from build123d import *

# Parameters (mm, degrees)
F1_DEPTH = 63.5
F2_DEPTH = 25.4
F3_DEPTH = 7.9375
F5_R     = 6.35
F6_R     = 9.6111188935
F7_DEPTH = 85.726


with BuildPart() as f1:
    # F0 (on Front) → F1 (new body, symmetric)
    with BuildSketch(Plane.XZ):
        Polygon((-41.275, 9.525), (-41.275, -9.525), (41.275, -9.525), (41.275, 9.525), (22.225, 9.525), align=None)
    extrude(amount=F1_DEPTH, both=True)

    # F0 (on Front) → F2 (join, symmetric)
    with BuildSketch(Plane.XZ):
        with BuildLine():
            Line((22.225, 9.525), (41.275, 9.525))
            Line((41.275, 9.525), (41.275, 36.5252))
            ThreePointArc((41.275, 36.5252), (45.9246798487, 47.7505201513), (57.15, 52.4002))
            Line((57.15, 52.4002), (60.325, 52.4002))
            Line((60.325, 52.4002), (60.325, 71.4502))
            Line((60.325, 71.4502), (57.15, 71.4502))
            add(Edge.make_bspline(
                [(53.2220163185, 71.2286086107), (54.5371358708, 71.3237902727), (55.8469463929, 71.3977482988), (57.15, 71.4502)],
                knots=[112.6539740509, 112.6539740509, 112.6539740509, 112.6539740509, 116.2850421165, 116.2850421165, 116.2850421165, 116.2850421165], degree=3))
            ThreePointArc((53.2220163185, 71.2286086107), (31.1025389426, 59.790740988), (22.225, 36.5252))
            Line((22.225, 36.5252), (22.225, 9.525))
        make_face()
        Polygon((85.725, 71.4502), (60.325, 71.4502), (60.325, 52.4002), (85.725, 52.4002), (85.725, 61.9125), align=None)
    extrude(amount=F2_DEPTH, both=True)

    # F0 (on Front) → F3 (join, symmetric)
    with BuildSketch(Plane.XZ):
        with BuildLine():
            add(Edge.make_bspline(
                [(-41.275, 9.525), (-33.4914332719, 44.8937261862), (12.4204005857, 68.2755952564), (53.2220163185, 71.2286086107)],
                knots=[0, 0, 0, 0, 112.6539740509, 112.6539740509, 112.6539740509, 112.6539740509], degree=3))
            Line((-41.275, 9.525), (22.225, 9.525))
            Line((22.225, 9.525), (22.225, 36.5252))
            ThreePointArc((22.225, 36.5252), (31.1025389426, 59.790740988), (53.2220163185, 71.2286086107))
        make_face()
    extrude(amount=F3_DEPTH, both=True)

    # F0 (on Front) → F4 (revolve)
    with BuildSketch(Plane.XZ):
        Polygon((85.725, 76.2), (85.725, 71.4502), (85.725, 61.9125), (85.725, 52.4002), (85.725, 47.625), (111.125, 47.625), (111.125, 76.2), align=None)
    revolve(axis=Axis((85.725, 0, 69.05625), (0, 0, 1)))

    # F5
    f5_edges = [f1.edges().sort_by_distance(p)[0] for p in [
        (41.275, -63.5, 0),
        (-41.275, -63.5, 0),
        (41.275, 63.5, 0),
        (-41.275, 63.5, 0),
    ]]
    fillet(f5_edges, radius=F5_R)

    # F6 (on face) → F7 (cut, through all)
    with BuildSketch(Plane.XY.offset(76.2)):
        with Locations((85.725, 0)):
            Circle(F6_R)
    extrude(amount=-F7_DEPTH, mode=Mode.SUBTRACT)


solid = f1.part
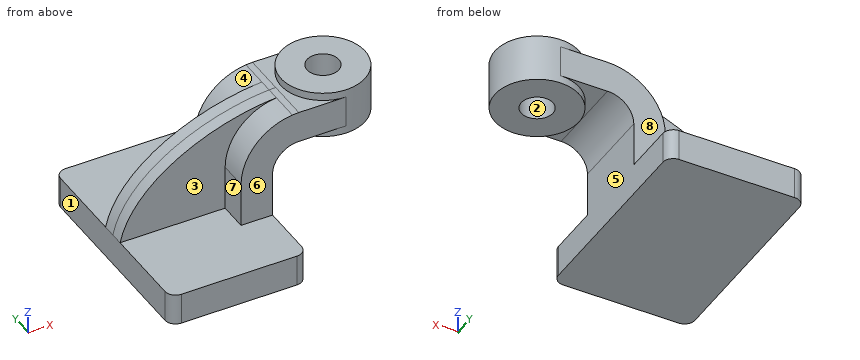
Verification items for the finished model (mm, model axes). Face numbers are marked on the shaded views. A direction names the side the tool comes from. Round coordinates to 2 decimals unless told otherwise and drop trailing zeros. Write each loop counter-clockwise with the first axis right and the second up, starting at its lowest first coordinate (ties: lowest second). Pieces come first, ordered by that corner, then holes.
(1) Depth check by flat-ended pin: pin 1 Ø5 at (x, z) = (29.5, 38) entering from -Y; pin 2 Ø2 at (x, z) = (1, 48) entering from -Y; pin 3 Ø5 at (y, z) = (-28.5, 46) entering from +X; pin 4 Ø18.5 at (x, z) = (28, 34) entering from +Y. Enter the tip coordinate at first touch or a pass-through.
Returned:
pin 1: stops at y = -25.4
pin 2: stops at y = -7.94
pin 3: passes through
pin 4: stops at y = 25.4
(2) Section check B-B (z = 5.5). Enter the section's corners in (x, y) (3 decimals), plus the area to 3 significant figures.
Returned:
outline: (-41.275, -57.15) arc R6.35 ccw to (-34.925, -63.5) - (34.925, -63.5) arc R6.35 ccw to (41.275, -57.15) - (41.275, 57.15) arc R6.35 ccw to (34.925, 63.5) - (-34.925, 63.5) arc R6.35 ccw to (-41.275, 57.15) - close
area: 10,400 mm2
(3) Material ranges on line 1 (X direction, y = 2, z = 0) (3 decimals); line 2 (Y direction, x = -5, z = 52); line 3 (Z direction, x = 96, y = -14) (3 decimals), recorded low to high.
Returned:
line 1: x = -41.275 to 41.275
line 2: y = -7.94 to 7.94
line 3: z = 47.625 to 76.2
(4) Section check C-C (y = 47). Enter the section's corners in (x, z) (3 decimals).
Returned:
outline: (-41.275, -9.525) - (41.275, -9.525) - (41.275, 9.525) - (-41.275, 9.525) - close
(5) Mould release check, pull along X, two halves, no side actions. Record for the marked faces 1, 2 and 3: pulls with the +X half, pulls with the -X half, needs draft (parallel to the pull), parting line crosses it, or undercut.
Returned:
face 1: pulls with the -X half
face 2: undercut
face 3: needs draft
(6) Access from +Z, -Z, +X, -X, +Y, -Y to the whole of each face (thin tool, end or side, straight path). Record for the marked faces 4, 5, 6, 7 and 8.
Returned:
face 4: +Z, -X, +Y
face 5: -Z, +X, +Y, -Y
face 6: +Z, +X, -X, -Y
face 7: +Z, -X, -Y
face 8: +Z, +X, -X, +Y
(7) Section check A-A (x = 81). Enter the section's corners in (y, z) (3 decimals), plus the area to 3 significant figures.
Returned:
outline: (-25.4, 52.4) - (-24.957, 52.4) - (-24.957, 47.625) - (-8.369, 47.625) - (-8.369, 76.2) - (-24.957, 76.2) - (-24.957, 71.45) - (-25.4, 71.45) - close; (8.369, 47.625) - (24.957, 47.625) - (24.957, 52.4) - (25.4, 52.4) - (25.4, 71.45) - (24.957, 71.45) - (24.957, 76.2) - (8.369, 76.2) - close
area: 965 mm2
